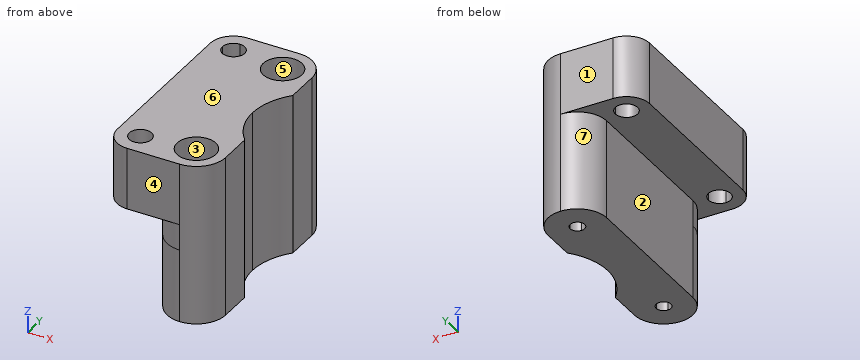
from build123d import *

# Parameters (mm, degrees)
F1_DEPTH = 15
F2_R     = 3.96875
F3_DEPTH = 18.02
F4_R     = 6.002975
F5_R     = 4.7625
F7_DEPTH = 33.02
F8_DEPTH = 5.32


# Not quite as in the source:
# - a fillet or chamfer is up to 0.001 mm smaller than in the source, because OpenCascade refuses the exact size


with BuildPart() as f1:
    # F0 (on Top) → F1 (new body)
    with BuildSketch(Plane.XY):
        Polygon((6.0029852, 0), (0, 0), (0, -43.0059592), (6.0029852, -43.0059592), (12.0059704, -43.0059592), (12.0059704, 0), align=None)
        with BuildLine():
            ThreePointArc((7.5029852, -37.002974), (7.0636453718, -38.0636341718), (6.0029852, -38.502974))
            ThreePointArc((6.0029852, -38.502974), (4.5029852, -37.002974), (6.0029852, -35.502974))
            ThreePointArc((6.0029852, -35.502974), (7.0636453718, -35.9423138282), (7.5029852, -37.002974))
        make_face(mode=Mode.SUBTRACT)
        with BuildLine():
            ThreePointArc((6.0029852, -7.5029852), (4.5029852, -6.0029852), (6.0029852, -4.5029852))
            ThreePointArc((6.0029852, -4.5029852), (7.0636453718, -4.9423250282), (7.5029852, -6.0029852))
            ThreePointArc((7.5029852, -6.0029852), (7.0636453718, -7.0636453718), (6.0029852, -7.5029852))
        make_face(mode=Mode.SUBTRACT)
    extrude(amount=F1_DEPTH)

    # F2 (on face) → F3 (join)
    with BuildSketch(Plane.XY.offset(15)):
        with BuildLine():
            Line((12.0059704, -43.0059592), (12.0059704, 0))
            Line((12.0059704, 0), (-4.7625, 0))
            Line((-4.7625, 0), (-4.7625, -2.4765))
            ThreePointArc((-4.7625, -2.4765), (-3.1460538982, -3.1460538982), (-2.4765, -4.7625))
            ThreePointArc((-2.4765, -4.7625), (-4.7625, -7.0485), (-7.0485, -4.7625))
            Line((-7.0485, -4.7625), (-9.525, -4.7625))
            Line((-9.525, -4.7625), (-9.525, -43.0059592))
            Line((-9.525, -43.0059592), (-4.7625, -43.0059592))
            Line((-4.7625, -43.0059592), (12.0059704, -43.0059592))
        make_face()
        with BuildLine():
            ThreePointArc((-2.4765, -38.2434592), (-3.1460538982, -39.8599053018), (-4.7625, -40.5294592))
            ThreePointArc((-4.7625, -40.5294592), (-6.3789461018, -36.6270130982), (-2.4765, -38.2434592))
        make_face(mode=Mode.SUBTRACT)
        with Locations((6.0029852, -37.002974)):
            Circle(F2_R, mode=Mode.SUBTRACT)
        with Locations((6.0029852, -6.0029852)):
            Circle(F2_R, mode=Mode.SUBTRACT)
        with BuildLine():
            Line((-4.7625, -2.4765), (-4.7625, 0))
            Line((-4.7625, 0), (-9.525, 0))
            Line((-9.525, 0), (-9.525, -4.7625))
            Line((-9.525, -4.7625), (-7.0485, -4.7625))
            ThreePointArc((-7.0485, -4.7625), (-6.3789461018, -3.1460538982), (-4.7625, -2.4765))
        make_face()
    extrude(amount=F3_DEPTH)

    # F4 (radius 6.0029852 in the source; OpenCascade refuses exactly that, so slightly less here)
    f4_edges = [f1.edges().sort_by_distance(p)[0] for p in [
        (12.00597, 0, 16.51),
        (0, 0, 7.5),
        (0, -43.005959, 7.5),
        (12.00597, -43.005959, 16.51),
    ]]
    fillet(f4_edges, radius=F4_R)

    # F5
    f5_edges = [f1.edges().sort_by_distance(p)[0] for p in [
        (-9.525, -43.005959, 24.01),
        (-9.525, 0, 24.01),
    ]]
    fillet(f5_edges, radius=F5_R)

    # F6 (on face) → F7 (cut, through all)
    with BuildSketch(Plane(origin=(0, 0, 0), x_dir=(1, 0, 0), z_dir=(0, 0, -1))):
        with BuildLine():
            ThreePointArc((12.0059704, 30.145029001), (9.5274974569, 26.1361174223), (8.6624922, 21.5029796))
            Line((8.6624922, 21.5029796), (12.0059704, 21.5029796))
            Line((12.0059704, 21.5029796), (12.0059704, 30.145029001))
        make_face()
        with BuildLine():
            Line((12.0059704, 21.5029796), (8.6624922, 21.5029796))
            ThreePointArc((8.6624922, 21.5029796), (9.5274974569, 16.8698417777), (12.0059704, 12.860930199))
            Line((12.0059704, 12.860930199), (12.0059704, 21.5029796))
        make_face()
    extrude(amount=-F7_DEPTH, mode=Mode.SUBTRACT)

    # F8 (cut): a face of the model
    f8_faces = [f1.faces().sort_by_distance(p)[0] for p in [
        (-4.4215962699, -21.5029796, 15),
    ]]
    extrude(f8_faces, amount=-F8_DEPTH, mode=Mode.SUBTRACT)


solid = f1.part
Geometry: final body of the model. Coordinates: model frame, mm. Face numbers are marked on the shaded views. A direction names the side the tool comes from. Round coordinates to 2 decimals unless told otherwise and drop trailing zeros. Loops run counter-clockwise (first coordinate to the right, second up) from the corner with the lowest first, then second, coordinate; pieces in that order, holes last. Notation, with made-up numbers: (13, -28.75) -> (38, -28.75) arc R23 cw to (38, 7.25) -> close; hole circle Ø2 at (-38.5, 13.5). An arc over 180 degrees is marked (long way). One line per question, with ' | ' between items. Start each with the question number.
1. Contact query for flat-ended pins moving along their axis: pin 1 (1.5 mm diameter, centred on x = -5, y = -32, fed in from -Z); pin 2 (10 mm diameter, centred on y = -21.5, z = 8.5, fed in from +X); pin 3 (6 mm diameter, centred on y = -24, z = 5.5, fed in from -X). Output: stop coordinate, or through.
2. Section D-D on y = -32. Output: boundary loops of the cut face in (x, z) (3 decimals).
3. Line query: line 1 along Y through (x, z) = (-5, 27); line 2 along X through (y, z) = (-38, 28) (1 decimal); line 3 along Y through (x, z) = (4.75, 26). Output: solid intervals per line, ascending. Write a range as [from, to].
4. Section B-B on x = -4.25. Output: boundary loops of the cut face in (y, z), and give its area (3 significant figures).
5. Set-up query: the marked faces 5, 6 and 7. Return all of +Z, -Z, +X, -X, +Y, -Y with unobstructed straight access to the full face (end or side cutting, diameter ignored); none if empty.
6. Mould query, pull axis Y, two halves, no side actions, for the marked faces 1, 2, 3 and 4. Classes: pulls with the +Y half, pulls with the -Y half, needs draft (parallel to the pull), parting line crosses it, or undercut.
7. Section C-C on z = 8.5. Count the separate pieces of the cut face and the enclosed holes in it, and give its area (3 significant figures).
8. Section A-A on z = 22. Output: boundary loops of the cut face in (x, y) (1 decimal).
Returned:
1) pin 1: stops at z = 20.32 | pin 2: stops at x = 9.68 | pin 3: stops at x = 0
2) outline: (-9.525, 20.32) -> (0, 20.32) -> (0, 0) -> (12.006, 0) -> (12.006, 33.02) -> (-9.525, 33.02) -> close
3) line 1: y = [-43, -40.52], [-35.97, -7.04], [-2.49, -0.01] | line 2: x = [-9.5, -7], [-2.5, 2.2], [9.8, 11.9] | line 3: y = [-43.01, -40.77], [-33.24, -9.77], [-2.24, 0]
4) outline: (-43.01, 20.32) -> (-40.47, 20.32) -> (-40.47, 33.02) -> (-43.01, 33.02) -> close; (-36.02, 20.32) -> (-6.99, 20.32) -> (-6.99, 33.02) -> (-36.02, 33.02) -> close; (-2.53, 20.32) -> (0, 20.32) -> (0, 33.02) -> (-2.53, 33.02) -> close | area: 433 mm2
5) face 5: +Z | face 6: +Z, +X, -X, +Y, -Y | face 7: -Z, -X, +Y
6) face 1: pulls with the +Y half | face 2: needs draft | face 3: undercut | face 4: pulls with the -Y half
7) separate pieces: 1 | enclosed holes: 2 | area: 432 mm2
8) outline: (-9.5, -38.2) arc R4.8 ccw to (-4.8, -43) -> (6, -43) arc R6 ccw to (12, -37) -> (12, -30.1) arc R12.8 cw to (12, -12.9) -> (12, -6) arc R6 ccw to (6, 0) -> (-4.8, 0) arc R4.8 ccw to (-9.5, -4.8) -> close; hole circle Ø4.6 at (-4.8, -38.2); hole circle Ø4.6 at (-4.8, -4.8); hole circle Ø7.9 at (6, -37); hole circle Ø7.9 at (6, -6)
